from build123d import *

# Parameters (mm, degrees)
SKETCH1_R               = 4
SKETCH1_R_2             = 3
BOSS_EXTRUDE1_DEPTH     = 6.8
CHAMFER1_SIZE           = 0.2
CUT_EXTRUDE1_REACH      = 13.236
CUT_EXTRUDE1_END_RADIUS = 3
SKETCH2_R               = 2
CIRPATTERN1_COUNT       = 2
CIRPATTERN1_ANGLE       = 90


with BuildPart() as part:
    # Sketch1 → Boss-Extrude1 (new body)
    with BuildSketch(Plane.XY):
        Circle(SKETCH1_R)
        Circle(SKETCH1_R_2, mode=Mode.SUBTRACT)
    extrude(amount=BOSS_EXTRUDE1_DEPTH)

    # Chamfer1
    chamfer1_edges = [part.edges().sort_by_distance(p)[0] for p in [
        (-4, 0, 0),
        (-4, 0, 6.8),
        (-3, 0, 0),
        (-3, 0, 6.8),
    ]]
    chamfer(chamfer1_edges, length=CHAMFER1_SIZE)

    # Cut-Extrude1: up to this cylinder (the profile starts outside it)
    cut_extrude1_end = Plane(origin=(0, 0, 3.3), z_dir=(0, 0, -1)) * Cylinder(CUT_EXTRUDE1_END_RADIUS, 33.472, mode=Mode.PRIVATE)
    # Sketch2 → Cut-Extrude1 (cut, up to the surface)
    with BuildSketch(Plane(origin=(4, 0, 0), x_dir=(0, 0, -1), z_dir=(1, 0, 0)), mode=Mode.PRIVATE) as cut_extrude1_sk1:
        with Locations((-3.3, 0)):
            Circle(SKETCH2_R)
    cut_extrude1_tool1 = extrude(cut_extrude1_sk1.sketch, amount=-CUT_EXTRUDE1_REACH, mode=Mode.PRIVATE) - cut_extrude1_end
    cut_extrude1 = cut_extrude1_tool1.solids().sort_by_distance((4, 0, 3.3))[0]
    add(cut_extrude1, mode=Mode.SUBTRACT)

    # CirPattern1: Cut-Extrude1 ×2 about axis
    cirpattern1_axis = Axis((0, 0, 6.6), (0, 0, 1))
    for i in range(1, CIRPATTERN1_COUNT):
        add(cut_extrude1.rotate(cirpattern1_axis, i * CIRPATTERN1_ANGLE / (CIRPATTERN1_COUNT - 1)), mode=Mode.SUBTRACT)


solid = part.part
Work out the finished part from the listing and answer in its coordinate system (mm). A direction names the side the tool comes from. Give positions to 0.01 mm unless a question says otherwise; leave off trailing zeros. Write each loop counter-clockwise with the first axis right and the second up, starting at its lowest first coordinate (ties: lowest second). Pieces come first, ordered by that corner, then holes. Notation, with made-up numbers: (26.25, -29.5) - (57.25, -29.5) arc R5 cw to (57.25, -23.5) - close; hole circle Ø1 at (0, 48.5). An arc over 180 degrees is marked (long way). One line per item, written item: value. Start each with the question number.
1. For a pull along Y with two mould halves and no side action, classify faces 1 (the cylindrical face through (3.13, 0.601, 1.392)), 2 (the flat face through (-2, -3, 0)), 3 (the cylindrical face through (-3.2, -2.4, 3.4)) as +Y half, -Y half, draft (parallel to the pull), parting line (faces both ways), or undercut.
2. Find section A-A (y = 0). Write down the section's boundary in (x, z), then the cut area to 3 significant figures.
3. Given pin 1 (2 mm diameter, centred on x = 2, z = 2, fed in from -Y); pin 2 (1.5 mm diameter, centred on x = 0, z = 2, fed in from +Y); pin 3 (1.5 mm diameter, centred on x = -2, z = 5, fed in from +Y), each flat-ended and moving along its own axis, determine where each tip first touches the part or whether it passes through.
4. Find section C-C (z = 2.75). Write down the section's boundary in (x, y).
5. Consider probe 1 along Z at (x, y) = (3.5, 0); probe 2 along Y at (x, z) = (-2, 2); probe 3 along X at (y, z) = (0.5, 6.5). Determine where each line is inside the solid, lowest interval first.
6. For faces 4 (the cylindrical face through (-0.601, 3.131, 1.392)), 5 (the flat face through (-2, -3, 6.8)), determine the directions among +Z, -Z, +X, -X, +Y, -Y from which every point of the face is accessible in a straight line to the end or side of a thin tool.
7. Find section D-D (z = 1). Write down the section's boundary in (x, y).
Geometry results:
1. face 1: undercut
1. face 2: draft
1. face 3: parting line
2. outline: (-4, 0.2) - (-3.8, 0) - (-3.2, 0) - (-3, 0.2) - (-3, 6.6) - (-3.2, 6.8) - (-3.8, 6.8) - (-4, 6.6) - close; (3, 0.2) - (3.2, 0) - (3.8, 0) - (4, 0.2) - (4, 1.3) - (3, 1.3) - close; (3, 5.3) - (4, 5.3) - (4, 6.6) - (3.8, 6.8) - (3.2, 6.8) - (3, 6.6) - close
2. area: 9.44 mm2
3. pin 1: y = -3.87
3. pin 2: y = 4
3. pin 3: y = 3.8
4. outline: (-1.92, 2.3) - (-1.92, 3.51) arc R4 ccw (long way) to (3.51, -1.92) - (2.3, -1.92) arc R3 cw (long way) to start; (1.92, 2.3) arc R3 cw to (2.3, 1.92) - (3.51, 1.92) arc R4 ccw to (1.92, 3.51) - close
5. probe 1: 0 to 1.3, 5.3 to 6.8
5. probe 2: -3.46 to -2.24, 2.24 to 3.46
5. probe 3: -3.97 to -2.96, 2.96 to 3.97
6. face 4: +Y
6. face 5: +Z, +X, -X, +Y, -Y
7. outline: circle Ø8 at (0, 0); hole circle Ø6 at (0, 0)
